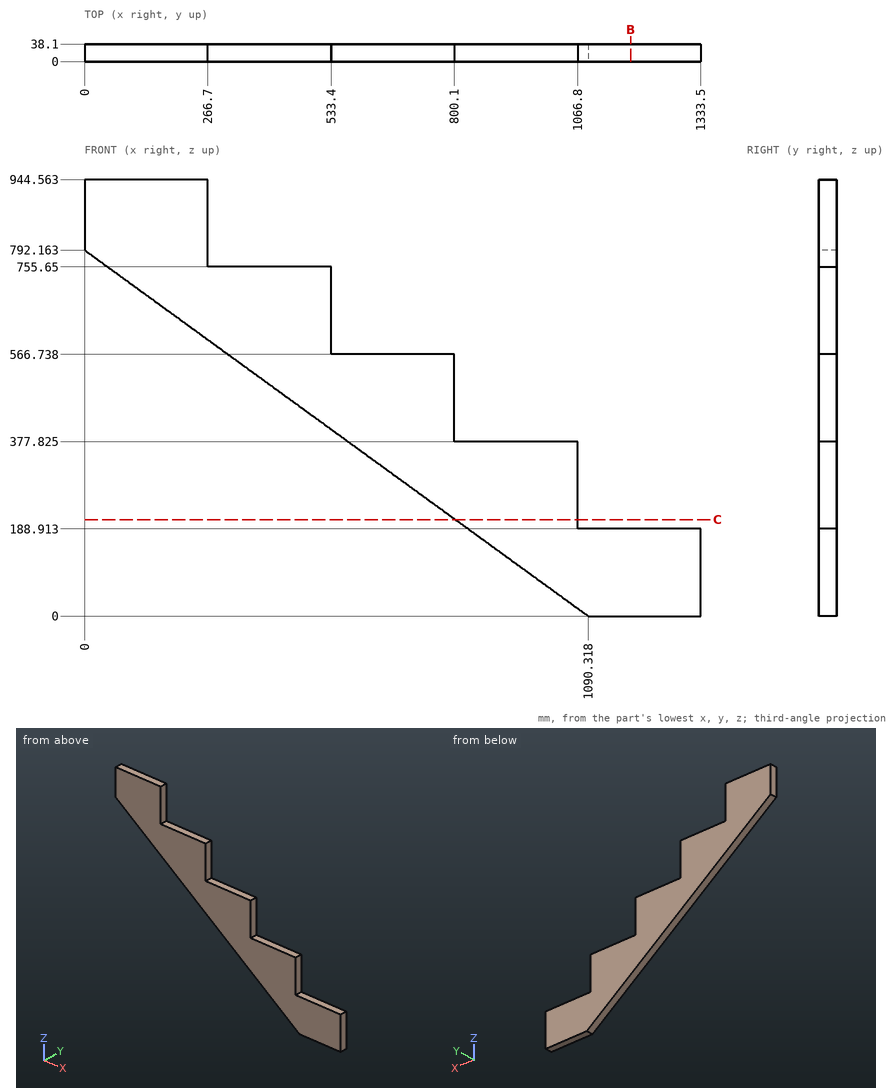
Job drawing, mm, ordinate dimensions from the low corner. One solid piece. Coordinates: 2 decimals unless noted, no trailing zeros. Write each loop counter-clockwise with the first axis right and the second up, starting at its lowest first coordinate (ties: lowest second). Pieces come first, ordered by that corner, then holes.
Item 1: Slice it at C-C (z = 209). Write the cut outline in (x, y) (1 decimal), and give its area (3 significant figures).
Item 2: Slice it at B-B (x = 1181.5). Write the cut outline in (y, z).
Item 3: Pin check, flat tips, straight feed: pin 1 (11.5 mm diameter, centred on y = 22, z = 830, fed in from +X); pin 2 (1 mm diameter, centred on y = 14.5, z = 464, fed in from +X); pin 3 (11.5 mm diameter, centred on x = 639, y = 26, fed in from +Z). Stop position of each tip, or through.
Item 4: Probe line 1 (Z direction, x = 1268, y = 8.5); line 2 (X direction, y = 34, z = 878); line 3 (Z direction, x = 255.5, y = 10). List the from-to ranges inside material, lowest first.
Results found:
1. outline: (802.7, 0) - (1066.8, 0) - (1066.8, 38.1) - (802.7, 38.1) - close
1. area: 10,100 mm2
2. outline: (0, 0) - (38.1, 0) - (38.1, 188.91) - (0, 188.91) - close
3. pin 1: stops at x = 266.7
3. pin 2: stops at x = 800.1
3. pin 3: stops at z = 566.74
4. line 1: z = 0 to 188.91
4. line 2: x = 0 to 266.7
4. line 3: z = 606.53 to 944.56
